from build123d import *

# Parameters (mm, degrees)
BOSS_EXTRUDE1_DEPTH     = 30
SKETCH2_W               = 36
SKETCH2_H               = 5
BOSS_EXTRUDE2_DEPTH     = 60
FILLET1_R               = 4
SKETCH4_W               = 20.656854249
SKETCH4_H               = 40
CUT_EXTRUDE1_DEPTH      = 31
CUT_EXTRUDE2_REACH      = 75.899
SKETCH3_R               = 8
CUT_EXTRUDE3_DEPTH      = 89.971905678
CUT_EXTRUDE3_DEPTH_BACK = 89.971905678


with BuildPart() as part:
    # Sketch1 → Boss-Extrude1 (new, symmetric)
    with BuildSketch(Plane.XY):
        with BuildLine():
            Line((10, 46), (-10, 46))
            Line((-10, 46), (-10, 35.656854249))
            ThreePointArc((-10, 35.656854249), (-10.30448187, 34.12612052), (-11.171572875, 32.828427125))
            Line((-11.171572875, 32.828427125), (-27.828427125, 16.171572875))
            ThreePointArc((-27.828427125, 16.171572875), (-29.12612052, 15.30448187), (-30.656854249, 15))
            Line((-30.656854249, 15), (-60, 15))
            Line((-60, 15), (-60, 0))
            Line((-60, 0), (60, 0))
            Line((60, 0), (60, 15))
            Line((60, 15), (30.656854249, 15))
            ThreePointArc((30.656854249, 15), (29.12612052, 15.30448187), (27.828427125, 16.171572875))
            Line((27.828427125, 16.171572875), (11.171572875, 32.828427125))
            ThreePointArc((11.171572875, 32.828427125), (10.30448187, 34.12612052), (10, 35.656854249))
            Line((10, 35.656854249), (10, 46))
        make_face()
    extrude(amount=BOSS_EXTRUDE1_DEPTH, both=True)

    # Sketch2 → Boss-Extrude2 (add, symmetric)
    with BuildSketch(Plane(origin=(0, 0, 0), x_dir=(0, 0, -1), z_dir=(1, 0, 0))):
        with Locations((0, -2.5)):
            Rectangle(SKETCH2_W, SKETCH2_H)
    extrude(amount=BOSS_EXTRUDE2_DEPTH, both=True)

    # Fillet1
    fillet1_edges = [part.edges().sort_by_distance(p)[0] for p in [
        (-60, 7.5, 30),
        (60, 7.5, -30),
        (-60, 7.5, -30),
        (60, 7.5, 30),
    ]]
    fillet(fillet1_edges, radius=FILLET1_R)

    # Sketch4 → Cut-Extrude1 (cut)
    with BuildSketch(Plane(origin=(0, 46, 0), x_dir=(1, 0, 0), z_dir=(0, 1, 0))):
        with Locations((-20.328427125, 0)):
            Rectangle(SKETCH4_W, SKETCH4_H)
    cut_extrude1 = extrude(amount=-CUT_EXTRUDE1_DEPTH, mode=Mode.SUBTRACT)

    # Sketch3 → Cut-Extrude2 (cut, up to next)
    with BuildSketch(Plane(origin=(0, 15, 0), x_dir=(1, 0, 0), z_dir=(0, 1, 0)), mode=Mode.PRIVATE) as cut_extrude2_sk1:
        with Locations(Location((-35, 0, 0), (0, 0, 180))):
            Circle(SKETCH3_R)
    cut_extrude2_tool1 = extrude(cut_extrude2_sk1.sketch, amount=-CUT_EXTRUDE2_REACH, mode=Mode.PRIVATE) & part.part
    cut_extrude2 = cut_extrude2_tool1.solids().sort_by_distance((-35, 15, 0))[0]
    add(cut_extrude2, mode=Mode.SUBTRACT)

    # Mirror1: Cut-Extrude1, Cut-Extrude2 across plane
    add(cut_extrude1.mirror(Plane(origin=(0, 0, 0), x_dir=(0, 0, 1), z_dir=(1, 0, 0))), mode=Mode.SUBTRACT)
    add(cut_extrude2.mirror(Plane(origin=(0, 0, 0), x_dir=(0, 0, 1), z_dir=(1, 0, 0))), mode=Mode.SUBTRACT)

    # Sketch5 → Cut-Extrude3 (cut, two sides: drawn at the far end of the back side and taken through both)
    with BuildSketch(Plane.ZY.offset(10).offset(-CUT_EXTRUDE3_DEPTH_BACK)):
        with BuildLine():
            Line((-20, 198.842570685), (-20, 46))
            ThreePointArc((-20, 46), (0, 26), (20, 46))
            Line((20, 46), (20, 198.842570685))
            Line((20, 198.842570685), (20, 504.527712056))
            Line((20, 504.527712056), (-20, 504.527712056))
            Line((-20, 504.527712056), (-20, 198.842570685))
        make_face()
    extrude(amount=CUT_EXTRUDE3_DEPTH + CUT_EXTRUDE3_DEPTH_BACK, mode=Mode.SUBTRACT)


solid = part.part
Design review of the part built by this model. Coordinates are the model's own, in mm. A direction names the side the tool comes from. Coordinates: 2 decimals unless noted, no trailing zeros. Loops run counter-clockwise (first coordinate to the right, second up) from the corner with the lowest first, then second, coordinate; pieces in that order, holes last. Notation, with made-up numbers: (-18.5, 14) -> (26.5, 14) arc R22 ccw to (26.5, 44) -> close; hole circle Ø11 at (87.5, 1). An arc over 180 degrees is marked (long way). Use a Markdown table: item, result. Add a question column.
Item 1: We need section A-A, the plane x = 35. Write out the cut boundary in (y, z).
Item 2: Clearance check with flat-ended pins moving along their axes: P1, Ø3, axis at y = 18, z = 16, coming from the -X side; P2, Ø3.5, axis at x = 1.5, z = -23.5, coming from the -Y side; P3, Ø4, axis at x = 8, y = -3.5, coming from the -Z side; P4, Ø10.5, axis at x = -22, y = 29.5, coming from the +Z side (3 decimals). State where each tip first meets the part, or that it passes through.
Item 3: We need section D-D, the plane x = -15. Write out the cut boundary in (y, z).
Item 4: Machinability: for faces 1 (the flat face through (1, -3, -18)), 2 (the flat face through (16, 21, 20)), 3 (the flat face through (-1, 0, 24)), 4 (the cylindrical face through (29.146, 15.296, 25.07)), 5 (the flat face through (-40, 15, 7)), which of the approach directions +Z, -Z, +X, -X, +Y, -Y give a long, thin tool a straight path to every point of the face, cutting with its end or side? Answer none if there is none.
Item 5: We need section C-C, the plane y = 42. Write out the cut boundary in (x, z), and give its area (3 significant figures).
Item 6: The part is to be moulded in two halves that separate along X. For faces 6 (the flat face through (-16, 21, -20)), 7 (the cylindrical face through (-28.651, 5.14, -4.868)), 8 (the cylindrical face through (-29.11, 15.31, 25.07)), say which applies: +X half, -X half, draft (parallel to the pull), parting line (faces both ways), or undercut.
Item 7: We need section B-B, the plane z = 0. Write out the cut boundary in (x, y).
Item 8: Wall thickness on L1, parallel to Z at x = -35, y = 3.25; L2, parallel to X at y = 7, z = 4; L3, parallel to Z at x = 35, y = -1: over which ranges is each line inside the solid? List them lowest first. Write a range as from..to.
Numbers:
| question | item | result |
|---|---|---|
| 1 | outline | (-5, -18) -> (0, -18) -> (0, -30) -> (15, -30) -> (15, -8) -> (-5, -8) -> close; (-5, 8) -> (15, 8) -> (15, 30) -> (0, 30) -> (0, 18) -> (-5, 18) -> close |
| 2 | P1 | stops at x = -10 |
| 2 | P2 | stops at y = 0 |
| 2 | P3 | stops at z = -18 |
| 2 | P4 | passes through |
| 3 | outline | (-5, -18) -> (0, -18) -> (0, -30) -> (29, -30) -> (29, -20) -> (15, -20) -> (15, 20) -> (29, 20) -> (29, 30) -> (0, 30) -> (0, 18) -> (-5, 18) -> close |
| 4 | face 1 | -Z, +X, -X, -Y |
| 4 | face 2 | +X, +Y |
| 4 | face 3 | +Z, +X, -X, -Y |
| 4 | face 4 | +Z, -Z, +X, +Y |
| 4 | face 5 | -X, +Y |
| 5 | outline | (-10, -30) -> (10, -30) -> (10, -19.6) -> (-10, -19.6) -> close; (-10, 19.6) -> (10, 19.6) -> (10, 30) -> (-10, 30) -> close |
| 5 | area | 416 mm^2 |
| 6 | face 6 | draft |
| 6 | face 7 | undercut |
| 6 | face 8 | -X half |
| 7 | outline | (-60, -5) -> (-43, -5) -> (-43, 15) -> (-60, 15) -> close; (-27, -5) -> (27, -5) -> (27, 15) -> (10, 15) -> (10, 26) -> (-10, 26) -> (-10, 15) -> (-27, 15) -> close; (43, -5) -> (60, -5) -> (60, 15) -> (43, 15) -> close |
| 8 | L1 | z = -30..-8, 8..30 |
| 8 | L2 | x = -60..-41.93, -28.07..28.07, 41.93..60 |
| 8 | L3 | z = -18..-8, 8..18 |
